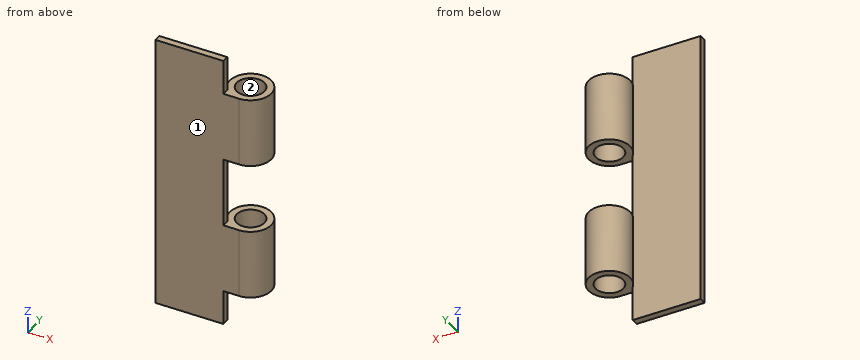
Autodesk Inventor part; units mm, degrees
ref_plane "Work Plane1" through (0, 0, -25) normal (0, 0, -1) x (-1, 0, 0)
ref_plane "YZ Plane" through (0, 0, 0) normal (1, 0, 0) x (0, 1, 0)
ref_plane "XZ Plane" through (0, 0, 0) normal (0, 1, 0) x (-1, 0, 0)
sketch "Sketch1" plane through (0, 0, 0) normal (0, 0, 1) x (1, 0, 0)
  line L0 (0, 0) -> (-12, 0)
  line L1 (-12, 0) -> (-12, 1)
  line L2 (-12, 1) -> (-2.2361, 1)
  arc A0 (0, 0) -> (-2.2361, 1) centre (0, 3) ccw
  circle A1 centre (0, 3) radius 2
  dimension "d1" = 1
  dimension "d2" = 4
  dimension "d3" = 12
  dimension "d4" = 3
  dimension "d5" = 1
  dimension "d6" = 3
extrude "Extrusion1" add sketch "Sketch1" against normal blind 40
sketch "Sketch2" plane through (0, 0, 0) normal (0, 0, 1) x (1, 0, 0)
  arc A0 (0, 0) -> (-2.2361, 1) centre (0, 3) ccw
  arc A1 (0, 0) -> (-2.2361, 1) centre (0, 3) ccw
  circle A2 centre (0, 3) radius 2
  circle A3 centre (0, 3) radius 2
  line L0 (-2.2361, 1) -> (-2.2361, 0)
  line L1 (-12, 0) -> (0, 0)
  line L2 (-2.2361, 0) -> (0, 0)
extrude "Extrusion2" cut sketch "Sketch2" against normal blind 5
sketch "Sketch3" plane through (0, 0, -40) normal (0, 0, -1) x (-1, 0, 0)
  arc A0 (2.2361, 1) -> (0, 0) centre (0, 3) ccw
  arc A1 (2.2361, 1) -> (0, 0) centre (0, 3) ccw
  circle A2 centre (0, 3) radius 2
  circle A3 centre (0, 3) radius 2
  line L0 (12, 1) -> (2.2361, 1)
  line L1 (2.2361, 1) -> (2.2361, 0)
  line L2 (0, 0) -> (12, 0)
  line L3 (2.2361, 0) -> (0, 0)
extrude "Extrusion3" cut sketch "Sketch3" against normal blind 5
ref_plane "Work Plane1" through (0, 0, -25) normal (0, 0, -1) x (-1, 0, 0)
sketch "Sketch4" plane through (0, 0, -25) normal (0, 0, -1) x (-1, 0, 0)
  arc A0 (2.2361, 1) -> (0, 0) centre (0, 3) ccw
  arc A1 (2.2361, 1) -> (0, 0) centre (0, 3) ccw
  circle A2 centre (0, 3) radius 2
  circle A3 centre (0, 3) radius 2
  line L0 (2.2361, 1) -> (2.2361, 0)
  line L1 (2.2361, 0) -> (0, 0)
  point P0 (0, 0)
extrude "Extrusion4" cut sketch "Sketch4" against normal blind 10
properties part number "Poker hinge 2"
The listing builds one solid part. Answer for the finished solid, in the listing's coordinates (mm). Face numbers are marked on the shaded views. Coordinates: 2 decimals unless noted, no trailing zeros. Write each loop counter-clockwise with the first axis right and the second up, starting at its lowest first coordinate (ties: lowest second). Pieces come first, ordered by that corner, then holes. Notation, with made-up numbers: M -15.75,51.25 L 5.25,51.25 A25 ccw 5.25,70.25 Z; hole C 51.5,2.25 d7. An arc over 180 degrees is marked long. Use a Markdown table: item, result. Add a question column.
1. Straight lines are drawn through the part: line 1 along Z through (x, y) = (-1.75, 0.5); line 2 along Y through (x, z) = (0, -7.25); line 3 along Y through (x, z) = (-9.75, -13.5). For each, find the intervals that lie inside material, in ascending order. Write a range as [from, to].
2. Given P1, Ø0.5, axis at y = 0.5, z = -3, coming from the +X side; P2, Ø8, axis at x = -9.5, z = -10, coming from the +Y side; P3, Ø1.8, axis at x = 0, y = 4.5, coming from the -Z side, each flat-ended and moving along its own axis, determine where each tip first touches the part or whether it passes through.
3. Section D-D (z = -3.5) is taken. Give the vertices of the cut face in (x, y), plus the area to 3 significant figures.
4. Section C-C (y = 5.5) is taken. Give the vertices of the cut face in (x, z), plus the area to 3 significant figures.
5. For a pull along X with two mould halves and no side action, classify the marked faces 1 and 2 as +X half, -X half, draft (parallel to the pull), parting line (faces both ways), or undercut.
6. Section A-A (y = 3) is taken. Give the vertices of the cut face in (x, z).
7. Section B-B (z = -32.5) is taken. Give the vertices of the cut face in (x, y), plus the area to 3 significant figures.
Data:
| question | item | result |
|---|---|---|
| 1 | line 1 | z = [-35, -25], [-15, -5] |
| 1 | line 2 | y = [0, 1], [5, 6] |
| 1 | line 3 | y = [0, 1] |
| 2 | P1 | stops at x = -2.24 |
| 2 | P2 | stops at y = 1 |
| 2 | P3 | stops at z = -35 |
| 3 | outline | M -12,0 L -2.24,0 L -2.24,1 L -12,1 Z |
| 3 | area | 9.76 mm2 |
| 4 | outline | M -1.66,-35 L 1.66,-35 L 1.66,-25 L -1.66,-25 Z; M -1.66,-15 L 1.66,-15 L 1.66,-5 L -1.66,-5 Z |
| 4 | area | 66.3 mm2 |
| 5 | face 1 | draft |
| 5 | face 2 | undercut |
| 6 | outline | M -3,-35 L -2,-35 L -2,-25 L -3,-25 Z; M -3,-15 L -2,-15 L -2,-5 L -3,-5 Z; M 2,-35 L 3,-35 L 3,-25 L 2,-25 Z; M 2,-15 L 3,-15 L 3,-5 L 2,-5 Z |
| 7 | outline | M -12,0 L 0,0 A3 ccw long -2.24,1 L -12,1 Z; hole C 0,3 d4 |
| 7 | area | 26.2 mm2 |
